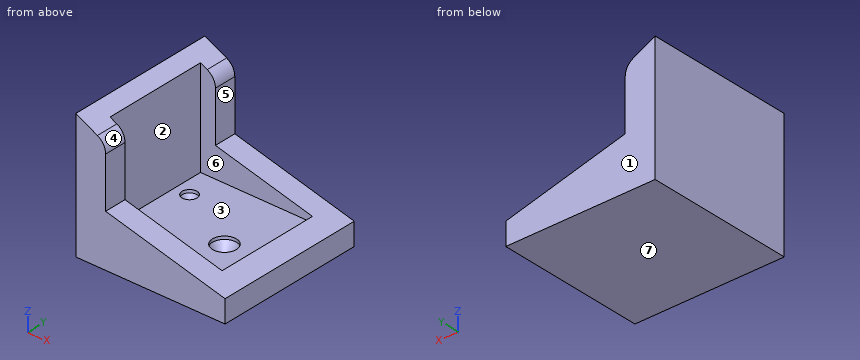
from build123d import *

# Parameters (mm, degrees)
F1_DEPTH  = 100
F2_R      = 9.9
F4_W      = 75
F4_H      = 70
F5_DEPTH  = 70.001
F6_R      = 5
F6_R_2    = 8
F7_DEPTH  = 8
F10_SIZE2 = 2.5
F10_SIZE  = 6
F11_SIZE2 = 3
F11_SIZE  = 6


with BuildPart() as f1:
    # F0 (on Front) → F1 (new body)
    with BuildSketch(Plane.XZ):
        Polygon((0, 85), (0, 0), (100, 0), (100, 15), (20, 35), (20, 75), align=None)
    extrude(amount=-F1_DEPTH)

    # F2
    f2_edges = [f1.edges().sort_by_distance(p)[0] for p in [
        (20, 50, 75),
    ]]
    fillet(f2_edges, radius=F2_R)

    # F4 (on offset) → F5 (cut, through all)
    with BuildSketch(Plane(origin=(0, 0, 15), x_dir=(1, 0, 0), z_dir=(0, 0, -1))):
        with Locations((47.5, -50)):
            Rectangle(F4_W, F4_H)
    extrude(amount=-F5_DEPTH, mode=Mode.SUBTRACT)

    # F6 (on face) → F7 (cut)
    with BuildSketch(Plane.XY.offset(15)):
        with Locations((20, 65)):
            Circle(F6_R)
        with Locations((65, 40)):
            Circle(F6_R_2)
    extrude(amount=-F7_DEPTH, mode=Mode.SUBTRACT)

    # F10
    f10_edges = [f1.edges().sort_by_distance(p)[0] for p in [
        (15, 65, 7),
    ]]
    f10_side = f1.faces().sort_by_distance((15, 65, 11))[0]
    chamfer(f10_edges, length=F10_SIZE, length2=F10_SIZE2, reference=f10_side)

    # F11
    f11_edges = [f1.edges().sort_by_distance(p)[0] for p in [
        (57, 40, 7),
    ]]
    f11_side = f1.faces().sort_by_distance((57, 40, 11))[0]
    chamfer(f11_edges, length=F11_SIZE, length2=F11_SIZE2, reference=f11_side)


solid = f1.part
Model file for the job. Use its own axes, mm. Face numbers are marked on the shaded views. A direction names the side the tool comes from. Give positions to 0.01 mm unless a question says otherwise; leave off trailing zeros. Order: outer loops, then holes, each group sorted by start corner. A loop starts at its lowest first (then second) coordinate and runs counter-clockwise, first axis right, second up. Notation, with made-up numbers: (83, 11) - (120, 11) arc R14 cw to (120, 37) - close; hole circle Ø10 at (6, 55.25). An arc over 180 degrees is marked (long way). One line per item, written item: value.
Item 1: Wall check: line 1 (Y direction, x = 15.5, z = 52); line 2 (Y direction, x = 20, z = 13.5); line 3 (Z direction, x = 15, y = 48.5). Give the ranges that are in metal, low to high.
Response values:
line 1: 0 to 15, 85 to 100
line 2: 0 to 60, 70 to 100
line 3: 0 to 15
Item 2: Two-plate mould, pull along Y, no slides. Class the marked faces 1, 2, 3 and 4: released by +Y, released by -Y, zero draft, split by the parting line, or undercut.
Response values:
face 1: released by +Y
face 2: undercut
face 3: undercut
face 4: zero draft
Item 3: Slice it at A-A (z = 46). List the corners of the cut face in (x, y), then the cut area to 3 significant figures.
Response values:
outline: (0, 0) - (20, 0) - (20, 15) - (10, 15) - (10, 85) - (20, 85) - (20, 100) - (0, 100) - close
area: 1,300 mm2
Item 4: Tool access for the marked faces 5, 6 and 7: list every direction of +Z, -Z, +X, -X, +Y, -Y with a clear straight run to the whole face (end or side of a thin tool).
Response values:
face 5: +Z, +X, +Y, -Y
face 6: +Z
face 7: -Z, +X, -X, +Y, -Y
Item 5: Pin check, flat tips, straight feed: pin 1 Ø1.5 at (x, y) = (41, 39.5) entering from +Z; pin 2 Ø8 at (x, y) = (67, 39.5) entering from +Z; pin 3 Ø10 at (x, z) = (47, 35) entering from +Y; pin 4 Ø4.5 at (y, z) = (6.5, 60) entering from +X. Stop position of each tip, or through.
Response values:
pin 1: z = 15
pin 2: z = 9.12
pin 3: through
pin 4: x = 20
Item 6: Slice it at D-D (y = 13). List the corners of the cut face in (x, z).
Response values:
outline: (0, 0) - (100, 0) - (100, 15) - (20, 35) - (20, 68.88) arc R9.9 ccw to (14.53, 77.74) - (0, 85) - close
Item 7: Slice it at B-B (x = 52). List the corners of the cut face in (y, z).
Response values:
outline: (0, 0) - (100, 0) - (100, 27) - (85, 27) - (85, 15) - (15, 15) - (15, 27) - (0, 27) - close
Item 8: Slice it at C-C (y = 40). List the corners of the cut face in (x, z), then the cut area to 3 significant figures.
Response values:
outline: (0, 0) - (100, 0) - (100, 15) - (85, 18.75) - (85, 15) - (73, 15) - (73, 13) - (70, 7) - (60, 7) - (57, 13) - (57, 15) - (10, 15) - (10, 80) - (0, 85) - close
area: 2,090 mm2
